Work out the finished part from the listing and answer in its coordinate system (mm). A direction names the side the tool comes from. Coordinates: 2 decimals unless noted, no trailing zeros. Loops run counter-clockwise (first coordinate to the right, second up) from the corner with the lowest first, then second, coordinate; pieces in that order, holes last.
```python
from build123d import *

# Parameters (mm, degrees)
CROQUIS1_W                  = 1.5
CROQUIS1_H                  = 13.7
SALIENTE_EXTRUIR1_DEPTH     = 14.7
REDONDEO1_R                 = 1
MATRIZL1_COUNT              = 3
MATRIZL1_PITCH              = 7.62
MATRIZL1_2_COUNT            = 3
MATRIZL1_2_PITCH            = 7.62
CROQUIS2_W                  = 31.98
CROQUIS2_H                  = 10.6
SALIENTE_EXTRUIR2_DEPTH     = 8.8
CROQUIS4_W                  = 1.2
CROQUIS4_H                  = 0.8
SALIENTE_EXTRUIR5_DEPTH     = 5
REDONDEO4_R                 = 0.5
MATRIZL2_COUNT              = 2
MATRIZL2_PITCH              = 7.62
REDONDEO4_OF_MATRIZL2_R     = 0.5
MATRIZL2_COL_COUNT          = 3
MATRIZL2_COL_PITCH          = 7.62
REDONDEO4_OF_MATRIZL2_COL_R = 0.5
CROQUIS5_W                  = 6.12
CROQUIS5_H                  = 8.6
SALIENTE_EXTRUIR6_DEPTH     = 0.5
CROQUIS6_W                  = 6.12
CROQUIS6_H                  = 6.6
SALIENTE_EXTRUIR7_DEPTH     = 1
CROQUIS7_R                  = 3
SALIENTE_EXTRUIR14_DEPTH    = 2
CORTAR_EXTRUIR2_START       = -1
CORTAR_EXTRUIR2_DEPTH       = 1
MATRIZL3_COUNT              = 2
MATRIZL3_PITCH              = 7.62
MATRIZL3_COL_COUNT          = 3
MATRIZL3_COL_PITCH          = 7.62


with BuildPart() as part:
    # Croquis1 → Saliente-Extruir1 (new body)
    with BuildSketch(Plane(origin=(0, 0, 0), x_dir=(1, 0, 0), z_dir=(0, 1, 0))):
        Rectangle(CROQUIS1_W, CROQUIS1_H)
    extrude(amount=SALIENTE_EXTRUIR1_DEPTH)

    # Redondeo1
    redondeo1_edges = [part.edges().sort_by_distance(p)[0] for p in [
        (0, 14.7, 6.85),
        (0, 14.7, -6.85),
    ]]
    fillet(redondeo1_edges, radius=REDONDEO1_R)


with BuildPart() as matrizl1_1:
    # MatrizL1: pattern copy
    add(part.part.moved(Location(Vector(1, 0, 0) * (1 * MATRIZL1_PITCH))))


with BuildPart() as matrizl1_2:
    # MatrizL1: pattern copy
    add(part.part.moved(Location(Vector(1, 0, 0) * (2 * MATRIZL1_PITCH))))


with BuildPart() as matrizl1_2_1:
    # MatrizL1 2: pattern copy
    add(part.part.moved(Location(Vector(-1, 0, 0) * (1 * MATRIZL1_2_PITCH))))


with BuildPart() as matrizl1_2_2:
    # MatrizL1 2: pattern copy
    add(part.part.moved(Location(Vector(-1, 0, 0) * (2 * MATRIZL1_2_PITCH))))


with BuildPart() as part_1:
    add(part.part)

    add(matrizl1_1.part)  # Saliente-Extruir2 merges MatrizL1_1

    add(matrizl1_2.part)  # Saliente-Extruir2 merges MatrizL1_2

    add(matrizl1_2_1.part)  # Saliente-Extruir2 merges MatrizL1 2_1

    add(matrizl1_2_2.part)  # Saliente-Extruir2 merges MatrizL1 2_2
    # Croquis2 → Saliente-Extruir2 (add)
    with BuildSketch(Plane(origin=(0, 0, 0), x_dir=(1, 0, 0), z_dir=(0, 1, 0))):
        Rectangle(CROQUIS2_W, CROQUIS2_H)
    extrude(amount=SALIENTE_EXTRUIR2_DEPTH)

    # Croquis4 → Saliente-Extruir5 (add)
    with BuildSketch(Plane.XZ):
        with Locations((-3.81, 0)):
            Rectangle(CROQUIS4_W, CROQUIS4_H)
    saliente_extruir5 = extrude(amount=SALIENTE_EXTRUIR5_DEPTH)

    # Redondeo4
    redondeo4_edges = [part_1.edges().sort_by_distance(p)[0] for p in [
        (-3.21, -5, 0),
        (-4.41, -5, 0),
    ]]
    fillet(redondeo4_edges, radius=REDONDEO4_R)

    # MatrizL2: Saliente-Extruir5 ×2
    with Locations(*[(-i * MATRIZL2_PITCH, 0, 0) for i in range(1, MATRIZL2_COUNT)]):
        add(saliente_extruir5)

    # Redondeo4 of MatrizL2
    redondeo4_of_matrizl2_edges = [part_1.edges().sort_by_distance(p)[0] for p in [
        (-10.83, -5, 0),
        (-12.03, -5, 0),
    ]]
    fillet(redondeo4_of_matrizl2_edges, radius=REDONDEO4_OF_MATRIZL2_R)

    # MatrizL2 col: Saliente-Extruir5 ×3
    with Locations(*[(i * MATRIZL2_COL_PITCH, 0, 0) for i in range(1, MATRIZL2_COL_COUNT)]):
        add(saliente_extruir5)

    # Redondeo4 of MatrizL2 col
    redondeo4_of_matrizl2_col_edges = [part_1.edges().sort_by_distance(p)[0] for p in [
        (4.41, -5, 0),
        (3.21, -5, 0),
        (12.03, -5, 0),
        (10.83, -5, 0),
    ]]
    fillet(redondeo4_of_matrizl2_col_edges, radius=REDONDEO4_OF_MATRIZL2_COL_R)

    # Croquis5 → Saliente-Extruir6 (add)
    with BuildSketch(Plane(origin=(0, 8.8, 0), x_dir=(1, 0, 0), z_dir=(0, 1, 0))):
        with Locations((-3.81, 0)):
            Rectangle(CROQUIS5_W, CROQUIS5_H)
    saliente_extruir6 = extrude(amount=SALIENTE_EXTRUIR6_DEPTH)

    # Croquis6 → Saliente-Extruir7 (add)
    with BuildSketch(Plane(origin=(0, 9.3, 0), x_dir=(1, 0, 0), z_dir=(0, 1, 0))):
        with Locations((-3.81, 0)):
            Rectangle(CROQUIS6_W, CROQUIS6_H)
    saliente_extruir7 = extrude(amount=SALIENTE_EXTRUIR7_DEPTH)

    # Croquis7 → Saliente-Extruir14 (add)
    with BuildSketch(Plane(origin=(0, 10.3, 0), x_dir=(1, 0, 0), z_dir=(0, 1, 0))):
        with Locations(Location((-3.81, 0, 0), (0, 0, 90))):
            Circle(CROQUIS7_R)
    saliente_extruir14 = extrude(amount=SALIENTE_EXTRUIR14_DEPTH)

    # Croquis13 → Cortar-Extruir2 (cut)
    with BuildSketch(Plane(origin=(0, 12.3, 0), x_dir=(1, 0, 0), z_dir=(0, 1, 0)).offset(CORTAR_EXTRUIR2_START)):
        with BuildLine():
            ThreePointArc((-5.548096676, 2.445203457), (-5.931320344, 2.121320344), (-6.255203457, 1.738096676))
            Line((-6.255203457, 1.738096676), (-4.517106781, 0))
            Line((-4.517106781, 0), (-3.81, 0.707106781))
            Line((-3.81, 0.707106781), (-5.548096676, 2.445203457))
        make_face()
        Polygon((-3.81, 0.707106781), (-3.102893219, 0), (-2.042233047, 1.060660172), (-2.749339828, 1.767766953), align=None)
        Polygon((-4.870660172, -1.767766953), (-3.81, -0.707106781), (-4.517106781, 0), (-5.577766953, -1.060660172), align=None)
        Polygon((-4.517106781, 0), (-3.81, -0.707106781), (-3.102893219, 0), (-3.81, 0.707106781), align=None)
        with BuildLine():
            Line((-3.81, -0.707106781), (-2.071903324, -2.445203457))
            ThreePointArc((-2.071903324, -2.445203457), (-1.688679656, -2.121320344), (-1.364796543, -1.738096676))
            Line((-1.364796543, -1.738096676), (-3.102893219, 0))
            Line((-3.102893219, 0), (-3.81, -0.707106781))
        make_face()
    cortar_extruir2 = extrude(amount=CORTAR_EXTRUIR2_DEPTH, mode=Mode.SUBTRACT)

    # MatrizL3: Saliente-Extruir6, Saliente-Extruir7, Saliente-Extruir14, Cortar-Extruir2 ×2
    with Locations(*[(-i * MATRIZL3_PITCH, 0, 0) for i in range(1, MATRIZL3_COUNT)]):
        add(saliente_extruir6)
        add(saliente_extruir7)
        add(saliente_extruir14)
        add(cortar_extruir2, mode=Mode.SUBTRACT)

    # MatrizL3 col: Saliente-Extruir6, Saliente-Extruir7, Saliente-Extruir14, Cortar-Extruir2 ×3
    with Locations(*[(i * MATRIZL3_COL_PITCH, 0, 0) for i in range(1, MATRIZL3_COL_COUNT)]):
        add(saliente_extruir6)
        add(saliente_extruir7)
        add(saliente_extruir14)
        add(cortar_extruir2, mode=Mode.SUBTRACT)


solid = part_1.part
```
1. For faces 1 (the flat face through (11, 9.3, 4)), 2 (the flat face through (13.018, 11.793, 0.881)), 3 (the flat face through (-4, -2, 0.4)), 4 (the flat face through (-4, 4, -5.3)), determine the directions among +Z, -Z, +X, -X, +Y, -Y from which every point of the face is accessible in a straight line to the end or side of a thin tool.
2. A cutting plane is placed at A-A, the plane y = -3. Give the vertices of the cut face in (x, z), then the cut area to 3 significant figures.
3. Determine the mould class of faces 5 (the flat face through (-8, 14.7, 0)), 6 (the flat face through (11, 4, 5.3)), 7 (the flat face through (-10.2, 11.793, -0.523)) for opening direction Z: released by +Z, released by -Z, zero draft, split by the parting line, or undercut.
4. Each of these flat-tipped pins is pushed along its axis until it touches: P1, Ø1.1, axis at x = -2.5, y = 9.5, coming from the +Z side; P2, Ø0.6, axis at x = -11, y = 9, coming from the +Z side; P3, Ø4, axis at x = -4, y = 7.5, coming from the -Z side. Where does it stop, or does it pass through?
5. Straight lines are drawn through the part: probe 1 along X at (y, z) = (12, -5); probe 2 along Y at (x, z) = (13.5, -1.25); probe 3 along Z at (x, y) = (12, 6). For each, find the intervals that lie inside material, in ascending order.
Answers below:
1. face 1: +Z, +Y
1. face 2: +Y
1. face 3: +Z, +X, -X, -Y
1. face 4: -Z, +Y, -Y
2. outline: (-12.03, -0.4) - (-10.83, -0.4) - (-10.83, 0.4) - (-12.03, 0.4) - close; (-4.41, -0.4) - (-3.21, -0.4) - (-3.21, 0.4) - (-4.41, 0.4) - close; (3.21, -0.4) - (4.41, -0.4) - (4.41, 0.4) - (3.21, 0.4) - close; (10.83, -0.4) - (12.03, -0.4) - (12.03, 0.4) - (10.83, 0.4) - close
2. area: 3.84 mm2
3. face 5: zero draft
3. face 6: released by +Z
3. face 7: undercut
4. P1: stops at z = 4.3
4. P2: stops at z = 5.3
4. P3: stops at z = -5.3
5. probe 1: x = -15.99 to -14.49, -8.37 to -6.87, -0.75 to 0.75, 6.87 to 8.37, 14.49 to 15.99
5. probe 2: y = 0 to 12.3
5. probe 3: z = -5.3 to 5.3
